The model under review builds one solid part; all positions refer to its coordinate system, in mm. A direction names the side the tool comes from. Round coordinates to 2 decimals unless told otherwise and drop trailing zeros. Order: outer loops, then holes, each group sorted by start corner. A loop starts at its lowest first (then second) coordinate and runs counter-clockwise, first axis right, second up. Notation, with made-up numbers: M -17.75,7.5 L 25.25,7.5 A38 ccw 25.25,45.5 Z; hole C -3,-24 d4. An arc over 180 degrees is marked long. Answer as a JSON object with one key per item and string values. Group by question number.
1. Mouldability with a two-part tool opening along X and no side actions: class faces 6 (the face through (19, 3.424, -17)), 7 (the face through (25.645, 2.461, 1.035)), 8 (the face through (23.849, 2.461, -9.485)) as released by +X, released by -X, zero draft, split by the parting line, or undercut.
2. To check wall thickness, follow probe 1 along X at (y, z) = (-0.15, 0); probe 2 along Z at (x, y) = (0, 0.3). State the ranges of each line that lie inside material, in increasing order. Write a range as [from, to].
3. Clearance check with flat-ended pins moving along their axes: P1, Ø2, axis at x = -0.5, y = 2, coming from the -Z side; P2, Ø0.6, axis at x = -0.5, y = 2.5, coming from the +Z side; P3, Ø1, axis at x = -10, y = 0.5, coming from the -Z side; P4, Ø14.5, axis at x = 10, z = 1, coming from the -Y side. State where each tip first meets the part, or that it passes through.
4. Add section A-A on x = 0. State the section outline as (y, z) points, and give its area (3 significant figures).
5. Machinability: for faces 1 (the face through (-15.89, 2.46, 21.82)), 2 (the face through (20.11, 2.461, -15.885)), 3 (the face through (-13.2, 0, -24.3)), 4 (the face through (-16.37, 2.46, 19.72)), 5 (the face through (-14.2, 2.46, 19.59)), which of the approach directions +Z, -Z, +X, -X, +Y, -Y give a long, thin tool a straight path to every point of the face, cutting with its end or side? Answer none if there is none.
6. Add section B-B on z = 0. State the section outline as (x, y) points.
Autodesk Inventor part; units mm, degrees
ref_plane "YZ Plane" through (0, 0, 0) normal (1, 0, 0) x (0, 1, 0)
ref_plane "XZ Plane" through (0, 0, 0) normal (0, 1, 0) x (-1, 0, 0)
ref_plane "XY Plane" through (0, 0, 0) normal (0, 0, 1) x (1, 0, 0)
sketch "Sketch1" plane through (0, 0, 0) normal (0, 1, 0) x (-1, 0, 0)
  circle A0 centre (0, 0) radius 21.9075
  circle A1 centre (0, 0) radius 29.972
  dimension "d0" = 59.944
  dimension "d1" = 43.815
extrude "Extrusion1" add sketch "Sketch1" along normal blind 1.524
sketch "Sketch2" plane through (0, 1.524, 0) normal (0, 1, 0) x (1, 0, 0)
  circle A0 centre (0, 0) radius 21.9075
  line L0 (-1.651, 24.1935) -> (1.651, 24.1935)
  line L1 (1.651, 24.1935) -> (1.651, 26.9935)
  line L2 (1.651, 26.9935) -> (-1.651, 26.9935)
  line L3 (-1.651, 26.9935) -> (-1.651, 24.1935)
  line L4 (-1.651, 24.1935) -> (1.651, 26.9935) construction
  line L5 (1.651, 24.1935) -> (-1.651, 26.9935) construction
  circle A1 centre (0, 0) radius 29.972
  point P0 (0, 25.5935)
  point P1 (0, 25.5935)
  dimension "d4" = 3.302
  dimension "d5" = 2.8
  dimension "d12" = 24.1935
extrude "Extrusion2" add sketch "Sketch2" along normal blind 1.9 contours L3 L2 L1 L0
pattern_circular "Circular Pattern1" count 15 over 360 about axis through (0, 0, 0) along (0, 1, 0) of "Extrusion2"
sketch "Sketch4" plane through (0, 0, 0) normal (1, 0, 0) x (0, 1, 0)
  line L0 (0, -27.432) -> (-0.3048, -27.432)
  line L1 (-0.3048, -27.432) -> (-0.3048, -24.257)
  line L2 (-0.3048, -24.257) -> (0, -24.257)
  line L3 (0, -24.257) -> (0, -27.432)
  line L4 (0, 29.972) -> (0, -29.972)
  line L5 (-1.0506, 0) -> (4.1698, 0)
  point P0 (0, 0)
  dimension "d21" = 3.175
  dimension "d22" = 0.3048
  dimension "d23" = 2.54
revolve "Revolution1" add sketch "Sketch4" angle 360 about axis through (0, -10, 0) along (0, 1, 0)
ref_plane "Work Plane1" through (-24.2026, 3.424, 12.0669) normal (-0.5, 0, -0.866) x (-0.866, 0, 0.5)
sketch "Sketch5" plane through (-24.2026, 3.424, 12.0669) normal (-0.5, 0, -0.866) x (-0.866, 0, 0.5)
  line L0 (-56.9655, -3.424) -> (2.9785, -3.424)
  line L1 (0.4385, -3.424) -> (-54.4255, -3.424)
  line L2 (2.6047, -3.424) -> (-4.6343, -3.424)
  line L3 (-4.6343, -3.424) -> (-4.6343, -4.694)
  line L4 (-4.6343, -4.694) -> (2.6047, -4.694)
  line L5 (2.6047, -4.694) -> (2.6047, -3.424)
  line L6 (-26.9935, -5.6328) -> (-26.9935, 0.9388)
  point P0 (-26.9935, -3.424)
  dimension "d25" = 1.27
  dimension "d26" = 0.3738
  dimension "d27" = 7.239
revolve "Revolution2" add sketch "Sketch5" angle 5 mid plane about axis through (-0.8255, -10, -1.4298) along (0, 1, 0)
properties part number "LEDRing"
Recorded:
{
 "1": {"face 6": "zero draft", "face 7": "released by +X", "face 8": "undercut"},
 "2": {"probe 1": "x = [-27.43, -24.26], [24.26, 27.43]", "probe 2": "z = [-29.97, -21.91], [21.91, 29.97]"},
 "3": {"P1": "stops at z = -29.97", "P2": "stops at z = -24.19", "P3": "stops at z = -28.43", "P4": "passes through"},
 "4": {"outline": "M -0.3,-27.43 L 0,-27.43 L 0,-29.97 L 1.52,-29.97 L 1.52,-26.99 L 3.42,-26.99 L 3.42,-24.19 L 1.52,-24.19 L 1.52,-21.91 L 0,-21.91 L 0,-24.26 L -0.3,-24.26 Z; M -0.3,24.26 L 0,24.26 L 0,21.91 L 1.52,21.91 L 1.52,29.97 L 0,29.97 L 0,27.43 L -0.3,27.43 Z", "area": "31.8 mm²"},
 "5": {"face 1": "+Z, -X, +Y", "face 2": "+X, +Y", "face 3": "-Y", "face 4": "-X, +Y", "face 5": "-Z, +Y"},
 "6": {"outline": "M -29.97,0 L -27.43,0 L -27.43,-0.3 L -24.26,-0.3 L -24.26,0 L -21.91,0 L -21.91,1.52 L -29.97,1.52 Z; M 21.91,0 L 24.26,0 L 24.26,-0.3 L 27.43,-0.3 L 27.43,0 L 29.97,0 L 29.97,1.52 L 21.91,1.52 Z"}
}
